Source: CAD feature listing. Evaluate the final solid. Frame: model axes, mm. Coordinates: 2 decimals unless noted, no trailing zeros. Order: outer loops, then holes, each group sorted by start corner. A loop starts at its lowest first (then second) coordinate and runs counter-clockwise, first axis right, second up.
Item 1: Section B-B on y = 0. Return the cut outline in (x, z), then the cut area to 3 significant figures.
Item 2: Ray query, line 1 (Y direction, x = 0, z = 1.5); line 2 (X direction, y = 21, z = -0.25); line 3 (Y direction, x = -9, z = 3.5). Return the intervals inside material, ascending.
Item 3: Section A-A on x = 0. Return the cut outline in (y, z), then the cut area to 3 significant figures.
Item 4: Section C-C on z = -2. State how many separate pieces and enclosed holes the cut face has, then the cut area to 3 significant figures.
from build123d import *

# Parameters (mm, degrees)
SKETCH1_W           = 200
SKETCH1_H           = 75
BOSS_EXTRUDE3_DEPTH = 5
SKETCH2_R           = 20
CUT_EXTRUDE1_DEPTH  = 155.939504323
CUT_EXTRUDE2_DEPTH  = 155.939504323
FILLET1_R           = 5


with BuildPart() as part:
    # Sketch1 → Boss-Extrude3 (new, symmetric)
    with BuildSketch(Plane.XY):
        with Locations((50, 0)):
            Rectangle(SKETCH1_W, SKETCH1_H)
    extrude(amount=BOSS_EXTRUDE3_DEPTH, both=True)

    # Sketch2 → Cut-Extrude1 (cut, through all)
    with BuildSketch(Plane.XY.offset(5)):
        Circle(SKETCH2_R)
    extrude(amount=-CUT_EXTRUDE1_DEPTH, mode=Mode.SUBTRACT)

    # Sketch3 → Cut-Extrude2 (cut, through all)
    with BuildSketch(Plane.XY.offset(5)):
        with BuildLine():
            Line((-43, 26.20895177), (-43, -26.20895177))
            Line((-43, -26.20895177), (-22.215366719, -11.466363047))
            ThreePointArc((-22.215366719, -11.466363047), (-25, 0), (-22.215366719, 11.466363047))
            Line((-22.215366719, 11.466363047), (-43, 26.20895177))
        make_face()
        with BuildLine():
            Line((-36.950325446, 30.5), (36.950325446, 30.5))
            Line((36.950325446, 30.5), (18.165562093, 17.175923668))
            ThreePointArc((18.165562093, 17.175923668), (0, 25), (-18.165562093, 17.175923668))
            Line((-18.165562093, 17.175923668), (-36.950325446, 30.5))
        make_face()
        with BuildLine():
            Line((22.215366719, 11.466363047), (43, 26.20895177))
            Line((43, 26.20895177), (43, -26.20895177))
            Line((43, -26.20895177), (22.215366719, -11.466363047))
            ThreePointArc((22.215366719, -11.466363047), (25, 0), (22.215366719, 11.466363047))
        make_face()
        with BuildLine():
            Line((-18.165562093, -17.175923668), (-36.950325446, -30.5))
            Line((-36.950325446, -30.5), (36.950325446, -30.5))
            Line((36.950325446, -30.5), (18.165562093, -17.175923668))
            ThreePointArc((18.165562093, -17.175923668), (0, -25), (-18.165562093, -17.175923668))
        make_face()
    extrude(amount=-CUT_EXTRUDE2_DEPTH, mode=Mode.SUBTRACT)

    # Fillet1
    fillet1_edges = [part.edges().sort_by_distance(p)[0] for p in [
        (-43, 26.20895177, 0),
        (-22.215366719, 11.466363047, 0),
        (-22.215366719, -11.466363047, 0),
        (-43, -26.20895177, 0),
        (-18.165562093, 17.175923668, 0),
        (-36.950325446, 30.5, 0),
        (36.950325446, 30.5, 0),
        (18.165562093, 17.175923668, 0),
        (22.215366719, -11.466363047, 0),
        (22.215366719, 11.466363047, 0),
        (43, 26.20895177, 0),
        (43, -26.20895177, 0),
        (-18.165562093, -17.175923668, 0),
        (18.165562093, -17.175923668, 0),
        (36.950325446, -30.5, 0),
        (-36.950325446, -30.5, 0),
    ]]
    fillet(fillet1_edges, radius=FILLET1_R)


solid = part.part
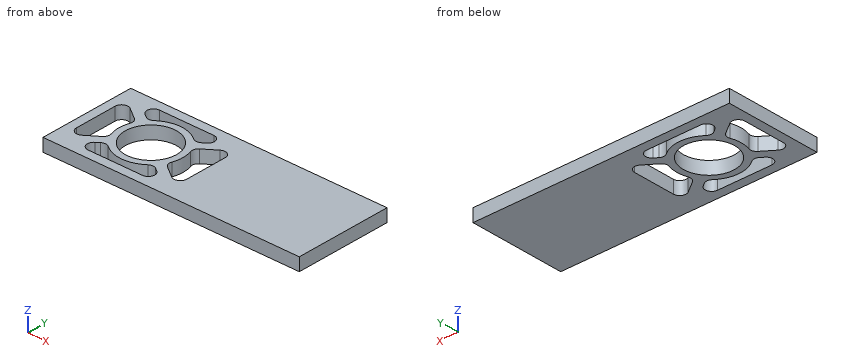
Answer list:
1. outline: (-50, -5) - (-43, -5) - (-43, 5) - (-50, 5) - close; (-25, -5) - (-20, -5) - (-20, 5) - (-25, 5) - close; (20, -5) - (25, -5) - (25, 5) - (20, 5) - close; (43, -5) - (150, -5) - (150, 5) - (43, 5) - close
1. area: 1,240 mm2
2. line 1: y = -37.5 to -30.5, -25 to -20, 20 to 25, 30.5 to 37.5
2. line 2: x = -50 to -40.25, -35.75 to -23.56, -13.56 to 13.56, 23.56 to 35.75, 40.25 to 150
2. line 3: y = -37.5 to -30.5, -23.32 to -17.86, 17.86 to 23.32, 30.5 to 37.5
3. outline: (-37.5, -5) - (-30.5, -5) - (-30.5, 5) - (-37.5, 5) - close; (-25, -5) - (-20, -5) - (-20, 5) - (-25, 5) - close; (20, -5) - (25, -5) - (25, 5) - (20, 5) - close; (30.5, -5) - (37.5, -5) - (37.5, 5) - (30.5, 5) - close
3. area: 240 mm2
4. separate pieces: 1
4. enclosed holes: 5
4. area: 11,500 mm2
